Read the model definition and answer for the solid it produces. Units are mm, in the model's axes. Face numbers are marked on the shaded views. A direction names the side the tool comes from. Give positions to 0.01 mm unless a question says otherwise; leave off trailing zeros. Loops run counter-clockwise (first coordinate to the right, second up) from the corner with the lowest first, then second, coordinate; pieces in that order, holes last. Notation, with made-up numbers: (6.5, 61) - (36.5, 61) arc R18 ccw to (36.5, 73) - close; hole circle Ø8 at (2, -29). An arc over 180 degrees is marked (long way). Use a Markdown table: item, result. Add a question column.
Item 1: A cutting plane is placed at D-D (z = -3.25). Determine the outline of the cut face in (x, y).
Item 2: A cutting plane is placed at C-C (z = -2.25). Determine the outline of the cut face in (x, y).
Item 3: A cutting plane is placed at A-A (x = 2.75). Determine the outline of the cut face in (y, z).
Item 4: Each of these flat-tipped pins is pushed along its axis until it touches: P1, Ø3, axis at x = 1, z = 1, coming from the +Y side; P2, Ø1.3, axis at x = 1, y = -3, coming from the +Z side; P3, Ø2, axis at y = -3.5, z = -1, coming from the -X side. Where does it stop, or does it pass through?
Item 5: A cutting plane is placed at B-B (y = -4). Determine the outline of the cut face in (x, z), plus the area to 3 significant figures.
Item 6: Which of the six approach directions +Z, -Z, +X, -X, +Y, -Y give full straight-line access (tool end or side, diameter ignored) to the marked faces 1, 2 and 3?
Item 7: Consider probe 1 along Z at (x, y) = (1.5, 0.75); probe 2 along Z at (x, y) = (1.5, -1.5). Determine where each line is inside the solid, lowest interval first. Write a range as [from, to].
from build123d import *

# Parameters (mm, degrees)
SKETCH1_R           = 2
BOSS_EXTRUDE1_DEPTH = 1.6
SKETCH1_3_W         = 8.2
SKETCH1_3_H         = 8.2
SKETCH1_3_W_2       = 6.2
SKETCH1_3_H_2       = 6.2
BOSS_EXTRUDE2_DEPTH = 2
BOSS_EXTRUDE3_START = -0.5
SKETCH1_4_W         = 8.2
SKETCH1_4_H         = 8.2
SKETCH1_4_W_2       = 6.2
SKETCH1_4_H_2       = 6.2
SKETCH1_4_R         = 2
BOSS_EXTRUDE3_DEPTH = 0.5
SKETCH3_W           = 5.8
SKETCH3_H           = 5.8
BOSS_EXTRUDE4_DEPTH = 4.5
CHAMFER1_SIZE       = 0.5
CUT_EXTRUDE1_DEPTH  = 0.2


with BuildPart() as part:
    # Sketch1 → Boss-Extrude1 (new body)
    with BuildSketch(Plane(origin=(0, 0, 0), x_dir=(1, 0, 0), z_dir=(0, 1, 0))):
        with Locations(Location((0, 0, 0), (0, 0, 270))):
            Circle(SKETCH1_R)
    extrude(amount=BOSS_EXTRUDE1_DEPTH)



with BuildPart() as body_2:
    # Sketch1_3 → Boss-Extrude2 (new body)
    with BuildSketch(Plane(origin=(0, 0, 0), x_dir=(1, 0, 0), z_dir=(0, 1, 0))):
        Rectangle(SKETCH1_3_W, SKETCH1_3_H)
        Rectangle(SKETCH1_3_W_2, SKETCH1_3_H_2, mode=Mode.SUBTRACT)
    extrude(amount=BOSS_EXTRUDE2_DEPTH)


with BuildPart() as part_1:
    add(part.part)

    add(body_2.part)  # Boss-Extrude3 merges body 2
    # Sketch1_4 → Boss-Extrude3 (add)
    # profile 1 of 3: a face of its own
    with BuildSketch(Plane(origin=(0, 0, 0), x_dir=(1, 0, 0), z_dir=(0, 1, 0)).offset(BOSS_EXTRUDE3_START)):
        Rectangle(SKETCH1_4_W, SKETCH1_4_H)
        Rectangle(SKETCH1_4_W_2, SKETCH1_4_H_2, mode=Mode.SUBTRACT)
    # profile 2 of 3: a face of its own
    with BuildSketch(Plane(origin=(0, 0, 0), x_dir=(1, 0, 0), z_dir=(0, 1, 0)).offset(BOSS_EXTRUDE3_START)):
        Rectangle(SKETCH1_4_W_2, SKETCH1_4_H_2)
        with Locations(Location((0, 0, 0), (0, 0, 270))):
            Circle(SKETCH1_4_R, mode=Mode.SUBTRACT)
    # profile 3 of 3: a face of its own
    with BuildSketch(Plane(origin=(0, 0, 0), x_dir=(1, 0, 0), z_dir=(0, 1, 0)).offset(BOSS_EXTRUDE3_START)):
        with Locations(Location((0, 0, 0), (0, 0, 270))):
            Circle(SKETCH1_4_R)
    extrude(amount=BOSS_EXTRUDE3_DEPTH)

    # Sketch3 → Boss-Extrude4 (add)
    with BuildSketch(Plane.XZ.offset(0.5)):
        Rectangle(SKETCH3_W, SKETCH3_H)
    extrude(amount=BOSS_EXTRUDE4_DEPTH)

    # Chamfer1
    chamfer1_edges = [part_1.edges().sort_by_distance(p)[0] for p in [
        (2.9, -2.75, -2.9),
        (2.9, -2.75, 2.9),
        (-2.9, -2.75, 2.9),
        (-2.9, -2.75, -2.9),
        (-4.1, 0.75, -4.1),
        (4.1, 0.75, -4.1),
        (4.1, 0.75, 4.1),
        (-4.1, 0.75, 4.1),
    ]]
    chamfer(chamfer1_edges, length=CHAMFER1_SIZE)

    # Sketch4 → Cut-Extrude1 (cut)
    with BuildSketch(Plane.XZ.offset(5)):
        with BuildLine():
            Line((1.673414591, 1.219479822), (1.398574847, 1.009143283))
            add(Edge.make_bspline(
                [(1.398574847, 1.009143283), (1.378968959, 1.032509253), (1.340021512, 1.078926169), (1.27736231, 1.144105713), (1.212060667, 1.205170975), (1.144141545, 1.262412854), (1.072382426, 1.31382962), (0.998521627, 1.362100723), (0.921323582, 1.405368461), (0.814571847, 1.457831447), (0.674923999, 1.512577602), (0.49912916, 1.558480834), (0.315618062, 1.587702009), (0.190420462, 1.590866851), (0.126739911, 1.592476617)],
                knots=[0, 0, 0, 0, 0.757959112, 1.505699292, 2.245454638, 2.979532153, 3.711538275, 4.438200793, 5.171680507, 5.909471876, 7.393775596, 8.890124382, 10.418191784, 12, 12, 12, 12], degree=3))
            add(Edge.make_bspline(
                [(0.126739911, 1.592476617), (0.091656612, 1.592072654), (0.021815619, 1.591268478), (-0.081832854, 1.580659353), (-0.183545905, 1.565748143), (-0.283257371, 1.54362282), (-0.38084033, 1.515650201), (-0.476932732, 1.482224787), (-0.570143332, 1.440869947), (-0.66176157, 1.395161687), (-0.749540781, 1.343534242), (-0.832595829, 1.28722089), (-0.910623797, 1.226851794), (-0.983686409, 1.162200688), (-1.051858357, 1.093558727), (-1.114645668, 1.020194386), (-1.171831078, 0.942342212), (-1.224548103, 0.861028804), (-1.271760837, 0.776491013), (-1.311290716, 0.688415942), (-1.346295838, 0.598311839), (-1.373995081, 0.505160679), (-1.395919598, 0.409617913), (-1.411047261, 0.311427125), (-1.421535732, 0.210793445), (-1.422335909, 0.142584133), (-1.422739255, 0.108201777)],
                knots=[0, 0, 0, 0, 1.054917814, 2.100044995, 3.131103042, 4.146048494, 5.169673617, 6.183595914, 7.203665975, 8.234915748, 9.262203917, 10.264457458, 11.251630812, 12.227803204, 13.197192746, 14.159520551, 15.12972552, 16.100847026, 17.073214652, 18.039054194, 19.002613845, 19.979014051, 20.95965708, 21.949030935, 22.966165397, 24, 24, 24, 24], degree=3))
            add(Edge.make_bspline(
                [(-1.422739255, 0.108201777), (-1.421477436, 0.056470457), (-1.419000022, -0.045097128), (-1.396951688, -0.193867738), (-1.363446597, -0.336388412), (-1.31323102, -0.471768254), (-1.251311969, -0.601676612), (-1.173071358, -0.723915466), (-1.08245482, -0.84033203), (-0.978180401, -0.948174978), (-0.863774585, -1.046688703), (-0.741026673, -1.133439285), (-0.610242385, -1.205754167), (-0.472865755, -1.265930114), (-0.327839641, -1.312186842), (-0.175424839, -1.344750965), (-0.015952844, -1.365993146), (0.093016556, -1.368026834), (0.148474687, -1.369061845)],
                knots=[0, 0, 0, 0, 1.029171465, 2.020641659, 2.987623507, 3.938342917, 4.889210282, 5.84687017, 6.821220943, 7.821438502, 8.827599549, 9.822697543, 10.807740252, 11.797342354, 12.80366471, 13.83203677, 14.896651826, 16, 16, 16, 16], degree=3))
            add(Edge.make_bspline(
                [(0.148474687, -1.369061845), (0.209577376, -1.367373065), (0.329842085, -1.364049143), (0.506210111, -1.335889893), (0.675045877, -1.290231976), (0.836358463, -1.226334053), (0.98969311, -1.143268765), (1.13528977, -1.042570888), (1.27327134, -0.923282555), (1.356242623, -0.832199427), (1.398574847, -0.785728511)],
                knots=[0, 0, 0, 0, 1.028121516, 2.023589091, 2.998037872, 3.967518031, 4.937445131, 5.927275754, 6.942489185, 8, 8, 8, 8], degree=3))
            Line((1.398574847, -0.785728511), (1.673414591, -0.993961685))
            add(Edge.make_bspline(
                [(1.673414591, -0.993961685), (1.651296481, -1.022500136), (1.607166206, -1.079440343), (1.535708189, -1.159712052), (1.460430891, -1.235216088), (1.380775181, -1.305343709), (1.29765739, -1.371498175), (1.209585077, -1.431800006), (1.117716045, -1.48709089), (1.022361566, -1.537717815), (0.923622953, -1.582635062), (0.821618518, -1.62108883), (0.716787943, -1.654213719), (0.609126434, -1.681465656), (0.498410678, -1.70273674), (0.385040203, -1.716956415), (0.268770328, -1.726698329), (0.190328907, -1.727586245), (0.150578052, -1.728036204)],
                knots=[0, 0, 0, 0, 0.986787822, 1.968848986, 2.935600012, 3.899624008, 4.868462664, 5.837806735, 6.815139263, 7.798259679, 8.787526145, 9.778297419, 10.776456485, 11.791383307, 12.812564526, 13.85620153, 14.913611965, 16, 16, 16, 16], degree=3))
            add(Edge.make_bspline(
                [(0.150578052, -1.728036204), (0.112934385, -1.727774211), (0.038498695, -1.727256153), (-0.071400056, -1.718863986), (-0.178389637, -1.707414249), (-0.282164263, -1.690174118), (-0.383290238, -1.669829778), (-0.480850823, -1.642558521), (-0.575806033, -1.612009355), (-0.667774374, -1.576104368), (-0.756834073, -1.535588185), (-0.842697885, -1.489796627), (-0.925326317, -1.439114762), (-1.005531738, -1.384659751), (-1.082129322, -1.32468245), (-1.155782847, -1.260015815), (-1.226905323, -1.190877804), (-1.270908008, -1.141022951), (-1.293031723, -1.115956877)],
                knots=[0, 0, 0, 0, 1.114604814, 2.203992996, 3.262667896, 4.300477797, 5.318619304, 6.316056647, 7.298880507, 8.271930387, 9.238335007, 10.195173496, 11.151986948, 12.108099108, 13.064862484, 14.031167946, 15.010108607, 16, 16, 16, 16], degree=3))
            add(Edge.make_bspline(
                [(-1.293031723, -1.115956877), (-1.328467367, -1.072415688), (-1.398910844, -0.985858978), (-1.489036527, -0.845572996), (-1.566184082, -0.699104787), (-1.628560003, -0.545684859), (-1.677322736, -0.385657471), (-1.711103931, -0.218941957), (-1.733055536, -0.045694015), (-1.735565825, 0.072142774), (-1.736841819, 0.132039918)],
                knots=[0, 0, 0, 0, 0.994628077, 1.977248131, 2.950237994, 3.925870899, 4.908910175, 5.911660606, 6.938484602, 8, 8, 8, 8], degree=3))
            add(Edge.make_bspline(
                [(-1.736841819, 0.132039918), (-1.735286626, 0.194995372), (-1.73222688, 0.318856296), (-1.706231084, 0.500630249), (-1.664412288, 0.674781648), (-1.605015399, 0.840985393), (-1.529710048, 1.000115673), (-1.436683434, 1.150956878), (-1.327016292, 1.294473678), (-1.201568724, 1.428488429), (-1.064001389, 1.551027782), (-0.916682575, 1.658833985), (-0.759900628, 1.748551501), (-0.595382776, 1.823547664), (-0.421897095, 1.881192127), (-0.239813726, 1.921545313), (-0.049474811, 1.94666243), (0.080387615, 1.949837638), (0.146371322, 1.951450976)],
                knots=[0, 0, 0, 0, 1.032925535, 2.032216505, 3.007276963, 3.968222605, 4.92396291, 5.891752235, 6.871517503, 7.883894988, 8.900124299, 9.891468569, 10.874487609, 11.85992873, 12.854644235, 13.869047385, 14.917252991, 16, 16, 16, 16], degree=3))
            add(Edge.make_bspline(
                [(0.146371322, 1.951450976), (0.186585794, 1.950968838), (0.266186291, 1.950014494), (0.383938943, 1.940708351), (0.49858127, 1.925194745), (0.610192252, 1.904078675), (0.719314868, 1.877871354), (0.825115109, 1.843731056), (0.928213796, 1.804694524), (1.027960704, 1.759736058), (1.123877255, 1.709269317), (1.215933573, 1.653853693), (1.303398432, 1.593557888), (1.38688728, 1.528894712), (1.465003491, 1.458496153), (1.53996497, 1.384298557), (1.609226048, 1.304164733), (1.651979243, 1.247759799), (1.673414591, 1.219479822)],
                knots=[0, 0, 0, 0, 1.096760587, 2.17092713, 3.219439832, 4.250915756, 5.268269357, 6.278326846, 7.281116186, 8.274029601, 9.260640565, 10.235837813, 11.203064059, 12.156899882, 13.114053108, 14.069676657, 15.032185724, 16, 16, 16, 16], degree=3))
        make_face()
    extrude(amount=-CUT_EXTRUDE1_DEPTH, mode=Mode.SUBTRACT)


solid = part_1.part
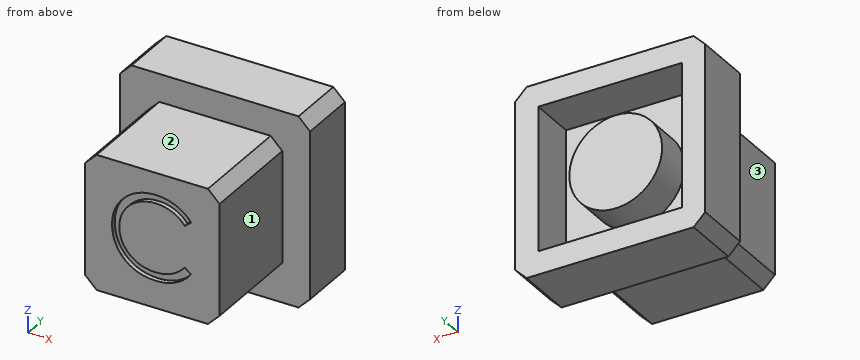
Geometry says:
| question | item | result |
|---|---|---|
| 1 | outline | (-4.1, -0.5) - (4.1, -0.5) - (4.1, 2) - (-4.1, 2) - close |
| 2 | outline | (-4.1, -0.5) - (-2.9, -0.5) - (-2.9, -5) - (2.9, -5) - (2.9, -0.5) - (4.1, -0.5) - (4.1, 2) - (3.1, 2) - (3.1, 0) - (-3.1, 0) - (-3.1, 2) - (-4.1, 2) - close |
| 3 | outline | (-5, -2.55) - (-0.5, -2.55) - (-0.5, -4.1) - (2, -4.1) - (2, -3.1) - (0, -3.1) - (0, 3.1) - (2, 3.1) - (2, 4.1) - (-0.5, 4.1) - (-0.5, 2.55) - (-5, 2.55) - close |
| 4 | P1 | y = 1.6 |
| 4 | P2 | z = 2.9 |
| 4 | P3 | x = -2.9 |
| 5 | outline | (-2.9, -2.4) - (-2.4, -2.9) - (2.4, -2.9) - (2.9, -2.4) - (2.9, 2.4) - (2.4, 2.9) - (-2.4, 2.9) - (-2.9, 2.4) - close |
| 5 | area | 33.1 mm² |
| 6 | face 1 | +Z, -Z, +X, -Y |
| 6 | face 2 | +Z, +X, -X, -Y |
| 6 | face 3 | +Z, -Z, -X, -Y |
| 7 | probe 1 | [-4.1, -3.1], [-1.32, 1.32], [3.1, 4.1] |
| 7 | probe 2 | [-2.9, 2.9] |
